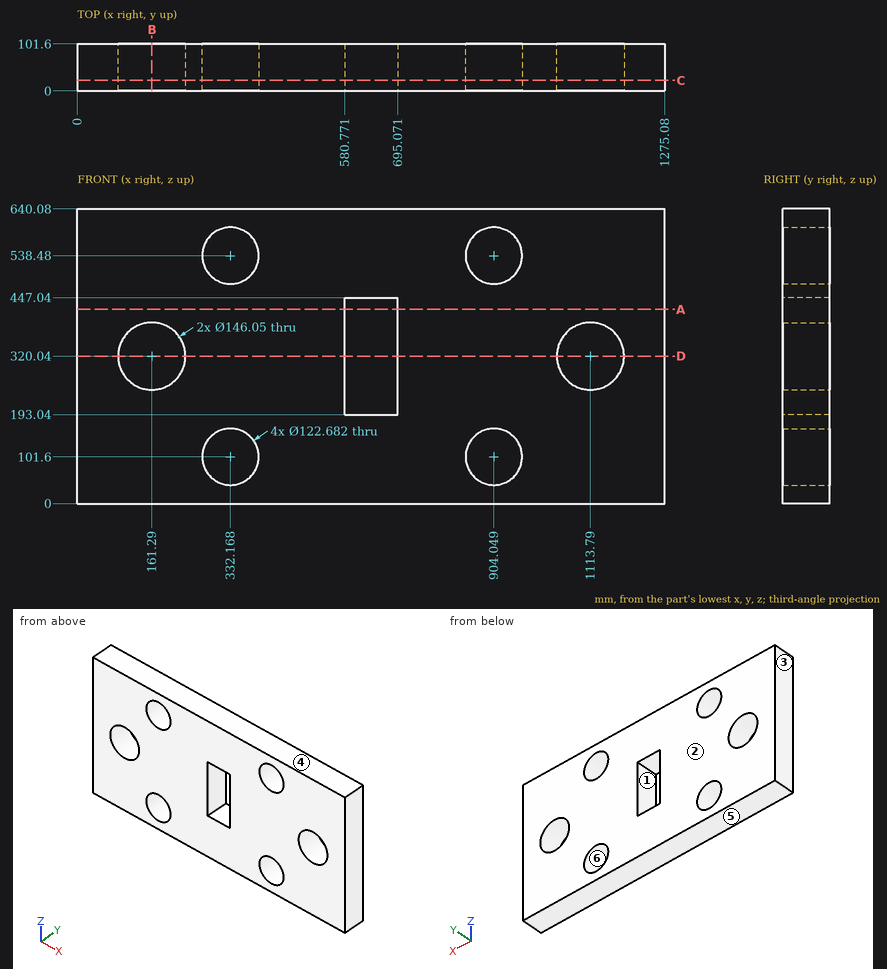
Answer from the drawing. Dimensions are ordinates in mm from the lowest x, y and z of the part. A direction names the side the tool comes from. Coordinates: 2 decimals unless noted, no trailing zeros. Write each loop counter-clockwise with the first axis right and the second up, starting at its lowest first coordinate (ties: lowest second). Pieces come first, ordered by that corner, then holes. Notation, with made-up numbers: (11.25, -12) - (53.25, -12) arc R5 ccw to (53.25, -5) - close; hole circle Ø5 at (-18, 36). An arc over 180 degrees is marked (long way). Answer as CSV lines item,"result".
1. Find section B-B (x = 161.29). Give the vertices of the cut face in (y, z) (1 decimal), plus the area to 3 significant figures.
Computed values:
outline,"(0, 0) - (101.6, 0) - (101.6, 247) - (0, 247) - close; (0, 393.1) - (101.6, 393.1) - (101.6, 640.1) - (0, 640.1) - close"
area,"50,200 mm²"
2. Find section D-D (z = 320.04). Give the vertices of the cut face in (x, y) (1 decimal), plus the area to 3 significant figures.
Computed values:
outline,"(0, 0) - (88.3, 0) - (88.3, 101.6) - (0, 101.6) - close; (234.3, 0) - (580.8, 0) - (580.8, 101.6) - (234.3, 101.6) - close; (695.1, 0) - (1040.8, 0) - (1040.8, 101.6) - (695.1, 101.6) - close; (1186.8, 0) - (1275.1, 0) - (1275.1, 101.6) - (1186.8, 101.6) - close"
area,"88,300 mm²"
3. Determine the mould class of the marked faces 3, 4, 5 and 6 for opening direction Z: +Z half, -Z half, draft (parallel to the pull), parting line (faces both ways), or undercut.
Computed values:
face 3,"draft"
face 4,"+Z half"
face 5,"-Z half"
face 6,"undercut"
4. A tool of negligible diameter and unlimited length cuts with its end or side. For the marked faces 1 and 2, from which of +Z, -Z, +X, -X, +Y, -Y can it reach the whole face along a straight path? Write none if from no direction.
Computed values:
face 1,"+Y, -Y"
face 2,"+Z, -Z, +X, -X, +Y"
5. Find section A-A (z = 421.5). Give the vertices of the cut face in (x, y), plus the area to 3 significant figures.
Computed values:
outline,"(0, 0) - (580.77, 0) - (580.77, 101.6) - (0, 101.6) - close; (695.07, 0) - (1275.08, 0) - (1275.08, 101.6) - (695.07, 101.6) - close"
area,"118,000 mm²"
6. Given P1, Ø4, axis at x = 1066.5, z = 106, coming from the -Y side, flat-ended and moving along its own axis, determine where the tip first touches the part or whether it passes through.
Computed values:
P1,"stops at y = 0"
7. Straight lines are drawn through the part: line 1 (X direction, y = 58, z = 101); line 2 (X direction, y = 84, z = 107) (1 decimal); line 3 (X direction, y = 54, z = 320) (1 decimal). For each, find the intervals that lie inside material, in ascending order. Write a range as [from, to].
Computed values:
line 1,"x = [0, 270.83], [393.51, 842.71], [965.39, 1275.08]"
line 2,"x = [0, 271.1], [393.3, 842.9], [965.2, 1275.1]"
line 3,"x = [0, 88.3], [234.3, 580.8], [695.1, 1040.8], [1186.8, 1275.1]"
8. Find section C-C (y = 22.5). Give the number of separate pieces and of enclosed holes in the cut face, plus the area to 3 significant figures.
Computed values:
separate pieces,"1"
enclosed holes,"7"
area,"706,000 mm²"
